Here's how the part is built. I have some questions about the finished solid (model axes, mm). A direction names the side the tool comes from. Give positions to 0.01 mm unless a question says otherwise; leave off trailing zeros. Loops run counter-clockwise (first coordinate to the right, second up) from the corner with the lowest first, then second, coordinate; pieces in that order, holes last. Notation, with made-up numbers: (14, 3) - (47, 3) arc R17 ccw to (47, 19) - close; hole circle Ø10 at (30, 45.25). An arc over 180 degrees is marked (long way). Use a Markdown table: item, result.
Autodesk Fusion 360 part; units mm, degrees
sketch "Sketch1" plane through (0, 0, 0) normal (1, 0, 0) x (0, 1, 0)
  line L0 (0, 0) -> (10, 0)
  line L1 (10, 0) -> (10, 45)
  line L2 (10, 55) -> (0, 55)
  line L3 (0, 55) -> (0, 0)
  line L4 (0, 55) -> (60, 55)
  line L5 (60, 55) -> (60, 45)
  line L6 (60, 45) -> (10, 45)
  line L7 (0, 45) -> (0, 55)
extrude "Extrude1" add sketch "Sketch1" along normal mid plane 100
sketch "Sketch2" plane through (0, 10, 0) normal (0, 1, 0) x (-1, 0, 0)
  line L0 (50, 45) -> (-50, 45)
  line L1 (-50, 45) -> (-50, 0)
  line L2 (-50, 0) -> (50, 0)
  line L3 (50, 0) -> (50, 45)
  circle A0 centre (25, 22.5) radius 3.75
  line L4 (0, 0) -> (0, 67.2521)
  circle A1 centre (-25, 22.5) radius 3.75
  dimension "d3" = 7.5
  dimension "d4" = 25
extrude "Extrude2" cut sketch "Sketch2" against normal blind 28 contours A0 | A1
sketch "Sketch3" plane through (0, 10, 0) normal (0, 1, 0) x (-1, 0, 0)
  circle A0 centre (-25, 22.5) radius 3.75
  circle A1 centre (25, 22.5) radius 3.75
  line L0 (50, 45) -> (-50, 45)
  line L1 (-50, 45) -> (-50, 0)
  line L2 (-50, 0) -> (50, 0)
  line L3 (50, 0) -> (50, 45)
  circle A2 centre (-25, 22.5) radius 5
  circle A3 centre (25, 22.5) radius 5
  dimension "d7" = 10
  dimension "d8" = 10
extrude "Extrude3" cut sketch "Sketch3" against normal blind 7.5 contours A2 | A3
fillet "Fillet1" radius 5 1 edges at (0, 10, 45)
chamfer "Chamfer1" distance 5 angle 45 1 edges at (0, 0, 55)
(1) We'd pull the mould along Z, two halves only. Please class faces 1 (the face through (23, 2.5, 26)), 2 (the face through (-1, 38, 45)), 3 (the face through (26.08, 6.3, 17.62)), 4 (the face through (-1, 60, 50)): pulls with the +Z half, pulls with the -Z half, needs draft (parallel to the pull), parting line crosses it, or undercut.
A:
| item | result |
|---|---|
| face 1 | undercut |
| face 2 | pulls with the -Z half |
| face 3 | undercut |
| face 4 | needs draft |
(2) Suppose I cut it at C-C on x = -37.5. Write out the boundary of the cut face in (y, z), plus the area to 3 significant figures.
A:
| item | result |
|---|---|
| outline | (0, 0) - (10, 0) - (10, 40) arc R5 cw to (15, 45) - (60, 45) - (60, 55) - (5, 55) - (0, 50) - close |
| area | 1,040 mm2 |
(3) Suppose I cut it at A-A on z = 22.5. Write out the boundary of the cut face in (x, y), plus the area to 4 significant figures.
A:
| item | result |
|---|---|
| outline | (-50, 0) - (-28.75, 0) - (-28.75, 2.5) - (-30, 2.5) - (-30, 10) - (-50, 10) - close; (-21.25, 0) - (21.25, 0) - (21.25, 2.5) - (20, 2.5) - (20, 10) - (-20, 10) - (-20, 2.5) - (-21.25, 2.5) - close; (28.75, 0) - (50, 0) - (50, 10) - (30, 10) - (30, 2.5) - (28.75, 2.5) - close |
| area | 812.5 mm2 |
(4) Suppose I cut it at D-D on y = 19. Write out the boundary of the cut face in (x, z), plus the area to 3 significant figures.
A:
| item | result |
|---|---|
| outline | (-50, 45) - (50, 45) - (50, 55) - (-50, 55) - close |
| area | 1,000 mm2 |
(5) Suppose I cut it at B-B on x = 25. Write out the boundary of the cut face in (y, z).
A:
| item | result |
|---|---|
| outline | (0, 0) - (10, 0) - (10, 17.5) - (2.5, 17.5) - (2.5, 18.75) - (0, 18.75) - close; (0, 26.25) - (2.5, 26.25) - (2.5, 27.5) - (10, 27.5) - (10, 40) arc R5 cw to (15, 45) - (60, 45) - (60, 55) - (5, 55) - (0, 50) - close |
(6) Will these pins go through, and if not, where does the flat tip stop? pin 1 (8 mm diameter, centred on x = -27, z = 20.5, fed in from +Y); pin 2 (8 mm diameter, centred on x = -38, y = 43.5, fed in from -Z); pin 3 (8.5 mm diameter, centred on x = 25, z = 22.5, fed in from +Y); pin 4 (16 mm diameter, centred on x = 25, z = 22.5, fed in from -Y).
A:
| item | result |
|---|---|
| pin 1 | y = 10 |
| pin 2 | z = 45 |
| pin 3 | y = 2.5 |
| pin 4 | y = 0 |
(7) If I drill on line 1 (Z direction, x = 25, y = 8); line 2 (Y direction, x = -20.5, z = 4.5); line 3 (Z direction, x = 25, y = 1.9), over which ranges is the centre line in solid material (lowest first)?
A:
| item | result |
|---|---|
| line 1 | 0 to 17.5, 27.5 to 55 |
| line 2 | 0 to 10 |
| line 3 | 0 to 18.75, 26.25 to 51.9 |
(8) On a 3-axis mill with a long thin cutter (end or side, diameter ignored), from which of +Z, -Z, +X, -X, +Y, -Y can I reach the whole of each face in a straight line? I mean faces 5 (the face through (-24.19, 1.27, 18.84)), 6 (the face through (-1, 10, 20)), 7 (the face through (-23.92, 6.3, 17.62)). Say none if no direction works.
A:
| item | result |
|---|---|
| face 5 | +Y, -Y |
| face 6 | -Z, +X, -X, +Y |
| face 7 | +Y |
